Geometry check sheet. Reference: the model listing, model coordinates, mm. A direction names the side the tool comes from. Give positions to 0.01 mm unless a question says otherwise; leave off trailing zeros. Loops run counter-clockwise (first coordinate to the right, second up) from the corner with the lowest first, then second, coordinate; pieces in that order, holes last. Notation, with made-up numbers: (69, -29) -> (101, -29) arc R10 cw to (101, -15) -> close; hole circle Ø11 at (-29, 37.25). An arc over 180 degrees is marked (long way). Answer as a JSON object with one key per item and string values.
from build123d import *

# Parameters (mm, degrees)
F1_DEPTH = 15
F3_DEPTH = 8.001
F5_D     = 4
F6_SIZE  = 5


with BuildPart() as f1:
    # F0 (on Front) → F1 (new body, symmetric)
    with BuildSketch(Plane.XZ):
        Polygon((0, 8), (0, 0), (46.2695387348, 0), (76.0110249394, -35.4445230334), (82.1393804843, -30.3022221559), (50, 8), align=None)
    extrude(amount=F1_DEPTH, both=True)

    # F2 (on Top) → F3 (cut, through all)
    with BuildSketch(Plane.XY):
        with BuildLine():
            ThreePointArc((15, 3), (12, 0), (15, -3))
            Line((15, -3), (35, -3))
            ThreePointArc((35, -3), (38, 0), (35, 3))
            Line((35, 3), (15, 3))
        make_face()
    extrude(amount=F3_DEPTH, mode=Mode.SUBTRACT)

    # F5 (through all)
    with Locations(Plane(origin=(33.2804354537, 0, 27.9256011146), x_dir=(0, 1, 0), z_dir=(0.7660444431, 0, 0.6427876097))):
        with Locations((0, -61.0110249394), (0, -41.0110249394)):
            Hole(F5_D / 2)

    # F6
    f6_edges = [f1.edges().sort_by_distance(p)[0] for p in [
        (0, 15, 4),
        (0, -15, 4),
    ]]
    chamfer(f6_edges, length=F6_SIZE)


solid = f1.part
1) Material ranges on line 1 along Z through (x, y) = (30.5, -12.25); line 2 along Y through (x, z) = (25, 5.5); line 3 along X through (y, z) = (11.75, -5), recorded low to high. Write a range as from..to.
Geometry check:
{"line 1": "z = 0..8", "line 2": "y = -15..-3, 3..15", "line 3": "x = 50.47..60.91"}
2) Section check D-D on z = -32.5. Record the cut outline in (x, y).
Geometry check:
{"outline": "(73.54, -15) -> (79.52, -15) -> (79.52, 15) -> (73.54, 15) -> close"}
3) Section check B-B on x = 45. Record the cut outline in (y, z), plus the area to 3 significant figures.
Geometry check:
{"outline": "(-15, 0) -> (15, 0) -> (15, 8) -> (-15, 8) -> close", "area": "240 mm2"}
4) Tool access check on faces 1 (the face through (3, -13, 4)), 2 (the face through (23, -4, 0)), 3 (the face through (38, 0, 4)). Record the directions out of +Z, -Z, +X, -X, +Y, -Y that give a thin tool (end or side, any length) a straight path to the whole face; none if there is none.
Geometry check:
{"face 1": "+Z, -Z, -X, -Y", "face 2": "-Z, -X, +Y, -Y", "face 3": "+Z, -Z"}
5) Section check A-A on y = 12.75. Record the cut outline in (x, z).
Geometry check:
{"outline": "(2.75, 0) -> (46.27, 0) -> (76.01, -35.44) -> (82.14, -30.3) -> (50, 8) -> (2.75, 8) -> close"}
6) Draft check along Z on faces 4 (the face through (69.883, -1.847, -22.006)), 5 (the face through (49, -15, -2)), 6 (the face through (79.03, -0.21, -32.91)). Enter one of: pulls with the +Z half, pulls with the -Z half, needs draft (parallel to the pull), parting line crosses it, or undercut.
Geometry check:
{"face 4": "undercut", "face 5": "needs draft", "face 6": "pulls with the -Z half"}
7) Depth check by flat-ended pin: P1, Ø1.5, axis at y = 12, z = -9, coming from the -X side; P2, Ø12, axis at y = -5.5, z = -14.5, coming from the -X side; P3, Ø1.5, axis at x = 11, z = -1, coming from the -Y side; P4, Ø15, axis at x = 22, y = 3.5, coming from the -Z side. Enter the tip coordinate at first touch or a pass-through.
Geometry check:
{"P1": "stops at x = 53.19", "P2": "stops at x = 53.4", "P3": "passes through", "P4": "stops at z = 0"}
8) Section check C-C on y = 0. Record the cut outline in (x, z), plus the area to 3 significant figures.
Geometry check:
{"outline": "(0, 0) -> (12, 0) -> (12, 8) -> (0, 8) -> close; (38, 0) -> (46.27, 0) -> (52.23, -7.1) -> (58.36, -1.96) -> (50, 8) -> (38, 8) -> close; (54.8, -10.17) -> (65.08, -22.42) -> (71.21, -17.28) -> (60.93, -5.02) -> close; (67.65, -25.49) -> (76.01, -35.44) -> (82.14, -30.3) -> (73.78, -20.34) -> close", "area": "498 mm2"}
